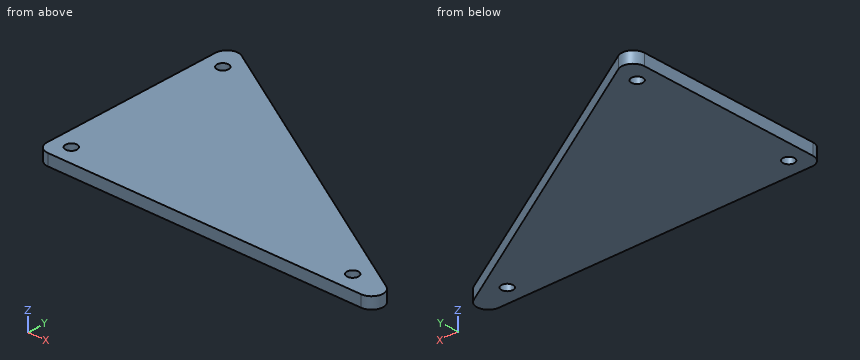
from build123d import *

# Parameters (mm, degrees)
ESBO_O1_R                = 2.5
RESSALTO_EXTRUS_O1_DEPTH = 5
FILETE1_R                = 5


with BuildPart() as part:
    # Esboço1 → Ressalto-extrusão1 (new body)
    with BuildSketch(Plane.XY):
        Polygon((80.424614017, -51.973967516), (-81.208731643, -51.973967516), (-81.208731643, 42.432853022), align=None)
        with Locations((-73.142213803, 28.456719531)):
            Circle(ESBO_O1_R, mode=Mode.SUBTRACT)
        with Locations((50.864750517, -43.973280469)):
            Circle(ESBO_O1_R, mode=Mode.SUBTRACT)
        with Locations((-73.275249483, -43.973280469)):
            Circle(ESBO_O1_R, mode=Mode.SUBTRACT)
    extrude(amount=RESSALTO_EXTRUS_O1_DEPTH)

    # Filete1
    filete1_edges = [part.edges().sort_by_distance(p)[0] for p in [
        (-81.208731643, 42.432853022, 2.5),
        (80.424614017, -51.973967516, 2.5),
        (-81.208731643, -51.973967516, 2.5),
    ]]
    fillet(filete1_edges, radius=FILETE1_R)


solid = part.part
Build history of the part. All positions in model axes, mm. Round coordinates to 2 decimals unless told otherwise and drop trailing zeros. Write each loop counter-clockwise with the first axis right and the second up, starting at its lowest first coordinate (ties: lowest second). Pieces come first, ordered by that corner, then holes. Notation, with made-up numbers: M 81,39.25 L 128,39.25 A18 cw 128,69.25 Z; hole C -33,-28 d6. An arc over 180 degrees is marked long. Answer in a Markdown table with one row per item.
1. Probe L1, parallel to Y at x = -73.5, z = 4.05; L2, parallel to Y at x = 50, z = 1.45; L3, parallel to Y at x = 48, z = 1.05. List the from-to ranges inside material, lowest first. Write a range as [from, to].
Geometry check:
| item | result |
|---|---|
| L1 | [-51.97, -46.46], [-41.48, 25.98], [30.93, 37.93] |
| L2 | [-51.97, -46.32], [-41.63, -34.2] |
| L3 | [-51.97, -33.04] |
2. Saw through at A-A (z = 4.05). List the corners of the cut face in (x, y).
Geometry check:
| item | result |
|---|---|
| outline | M -81.21,-46.97 A5 ccw -76.21,-51.97 L 61.95,-51.97 A5 ccw 64.47,-42.66 L -73.69,38.04 A5 ccw -81.21,33.72 Z; hole C -73.28,-43.97 d5; hole C -73.14,28.46 d5; hole C 50.86,-43.97 d5 |
3. Saw through at B-B (y = -0.5). List the corners of the cut face in (x, z), and give its area (3 significant figures).
Geometry check:
| item | result |
|---|---|
| outline | M -81.21,0 L -7.7,0 L -7.7,5 L -81.21,5 Z |
| area | 368 mm2 |
4. Saw through at C-C (x = 58.5). List the corners of the cut face in (y, z), and give its area (3 significant figures).
Geometry check:
| item | result |
|---|---|
| outline | M -51.97,0 L -39.17,0 L -39.17,5 L -51.97,5 Z |
| area | 64.0 mm2 |
